from build123d import *

# Parameters (mm, degrees)
SKETCH1_W            = 15
SKETCH1_H            = 7.3
BOSS_EXTRUDE1_DEPTH  = 1
SKETCH2_W            = 3.05
SKETCH2_H            = 2.36
CUT_EXTRUDE1_DEPTH   = 1
SKETCH5_W            = 1
SKETCH5_H            = 4.94
ENGTH_EXTRUDE_DEPTH  = 1.7874
SKETCH6_W            = 4.61
SKETCH6_H            = 1
HEIGHT_EXTRUDE_DEPTH = 1.7874
SCREWS_R             = 0.5
CUT_EXTRUDE2_DEPTH   = 1
SKETCH8_W            = 1
SKETCH8_H            = 1
PINS_DEPTH           = 1


with BuildPart() as part:
    # Sketch1 → Boss-Extrude1 (new body)
    with BuildSketch(Plane.XY):
        with Locations((88.072707455, -6.376080206)):
            Rectangle(SKETCH1_W, SKETCH1_H)
    extrude(amount=BOSS_EXTRUDE1_DEPTH)

    # Sketch2 → Cut-Extrude1 (cut)
    with BuildSketch(Plane.XY.offset(1)):
        with Locations((94.047707455, -3.906080206)):
            Rectangle(SKETCH2_W, SKETCH2_H)
    extrude(amount=-CUT_EXTRUDE1_DEPTH, mode=Mode.SUBTRACT)

    # Sketch5 → :ength-Extrude (add)
    with BuildSketch(Plane(origin=(95.572707455, 0, 0), x_dir=(0, 0, -1), z_dir=(1, 0, 0))):
        with Locations((-0.5, -7.556080206)):
            Rectangle(SKETCH5_W, SKETCH5_H)
    extrude(amount=ENGTH_EXTRUDE_DEPTH)

    # Sketch6 → Height-Extrude (add)
    with BuildSketch(Plane(origin=(0, -2.726080206, 0), x_dir=(1, 0, 0), z_dir=(0, 1, 0))):
        with Locations((90.217707455, -0.5)):
            Rectangle(SKETCH6_W, SKETCH6_H)
    extrude(amount=HEIGHT_EXTRUDE_DEPTH)

    # Screws → Cut-Extrude2 (cut)
    with BuildSketch(Plane(origin=(0, 0, 0), x_dir=(-1, 0, 0), z_dir=(0, 0, -1))):
        with Locations((-81.572707455, -7.026080206)):
            Circle(SCREWS_R)
        with Locations((-88.322707455, -10.026080206)):
            Circle(SCREWS_R)
        with Locations((-94.072707455, -6.026080206)):
            Circle(SCREWS_R)
    extrude(amount=-CUT_EXTRUDE2_DEPTH, mode=Mode.SUBTRACT)

    # Sketch8 → Pins (add)
    with BuildSketch(Plane(origin=(0, 0, 0), x_dir=(-1, 0, 0), z_dir=(0, 0, -1))):
        with Locations((-92.022707455, -1.438680206)):
            Rectangle(SKETCH8_W, SKETCH8_H)
        with Locations((-88.412707455, -1.438680206)):
            Rectangle(SKETCH8_W, SKETCH8_H)
        with Locations((-96.860107455, -5.586080206)):
            Rectangle(SKETCH8_W, SKETCH8_H)
        with Locations((-96.860107455, -9.526080206)):
            Rectangle(SKETCH8_W, SKETCH8_H)
    extrude(amount=PINS_DEPTH)


solid = part.part
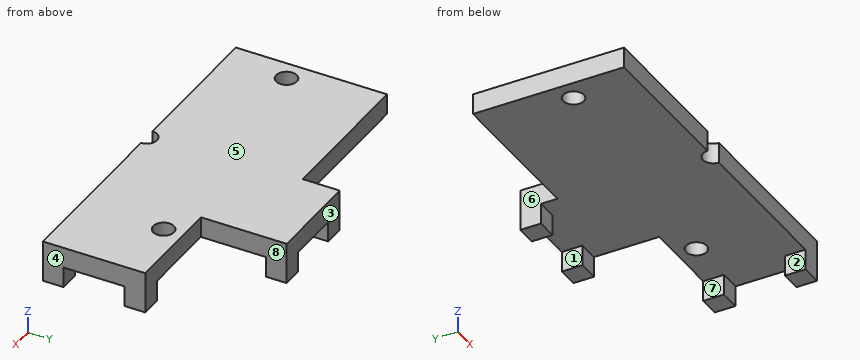
The model under review builds one solid part; all positions refer to its coordinate system, in mm. Face numbers are marked on the shaded views. A direction names the side the tool comes from. Coordinates: 2 decimals unless noted, no trailing zeros. Write each loop counter-clockwise with the first axis right and the second up, starting at its lowest first coordinate (ties: lowest second). Pieces come first, ordered by that corner, then holes. Notation, with made-up numbers: (31, -21) - (68, -21) arc R25 ccw to (68, 16) - close; hole circle Ø1 at (80, -23.75). An arc over 180 degrees is marked (long way). Answer as a JSON object with one key per item and string values. Group by question number.
1. Mouldability with a two-part tool opening along X and no side actions: class the marked faces 1, 2 and 3 as pulls with the +X half, pulls with the -X half, needs draft (parallel to the pull), parting line crosses it, or undercut.
2. Add section A-A (z = -0.3). Give the boundary of the cut face in (x, y), plus the area to 3 significant figures.
3. Add section B-B (y = -7.25). Give the boundary of the cut face in (x, z).
4. Add section D-D (x = 85). Give the boundary of the cut face in (y, z), plus the area to 3 significant figures.
5. Machinability: for the marked faces 4, 5, 6, 7 and 8, which of the approach directions +Z, -Z, +X, -X, +Y, -Y give a long, thin tool a straight path to every point of the face, cutting with its end or side? Answer none if there is none.
6. To check wall thickness, follow probe 1 along Y at (x, z) = (96.75, -0.5); probe 2 along Y at (x, z) = (86, 0.1); probe 3 along Z at (x, y) = (92.25, -3.5). State the ranges of each line that lie inside material, in increasing order.
7. Add section C-C (y = -1.5). Give the boundary of the cut face in (x, z), plus the area to 3 significant figures.
8. Clearance check with flat-ended pins moving along their axes: pin 1 Ø0.8 at (x, z) = (82.5, 0.5) entering from +Y; pin 2 Ø0.8 at (y, z) = (-5.5, -0.5) entering from -X; pin 3 Ø0.6 at (x, z) = (96, 0) entering from +Y. State where each tip first meets the part, or that it passes through.
Findings:
{
 "1": {"face 1": "undercut", "face 2": "pulls with the -X half", "face 3": "needs draft"},
 "2": {"outline": "(87.91, -1.94) - (88.91, -1.94) - (88.91, -0.94) - (87.91, -0.94) - close; (91.52, -1.94) - (92.52, -1.94) - (92.52, -0.94) - (91.52, -0.94) - close; (96.36, -10.03) - (97.36, -10.03) - (97.36, -9.03) - (96.36, -9.03) - close; (96.36, -6.09) - (97.36, -6.09) - (97.36, -5.09) - (96.36, -5.09) - close", "area": "4.00 mm²"},
 "3": {"outline": "(80.57, 0) - (81.13, 0) - (81.13, 1) - (80.57, 1) - close; (82.02, 0) - (97.36, 0) - (97.36, 1) - (82.02, 1) - close"},
 "4": {"outline": "(-10.03, 0) - (-2.73, 0) - (-2.73, 1) - (-10.03, 1) - close", "area": "7.30 mm²"},
 "5": {"face 4": "+Z, -Z, +X, +Y, -Y", "face 5": "+Z, +X, -X, +Y, -Y", "face 6": "+Z, -Z, -X, +Y", "face 7": "-Z, -X, +Y, -Y", "face 8": "+Z, -Z, +X, +Y"},
 "6": {"probe 1": "-10.03 to -9.03, -6.09 to -5.09", "probe 2": "-10.03 to -2.73", "probe 3": "0 to 1"},
 "7": {"outline": "(87.91, -1) - (88.91, -1) - (88.91, 0) - (91.52, 0) - (91.52, -1) - (92.52, -1) - (92.52, 1) - (87.91, 1) - close", "area": "6.61 mm²"},
 "8": {"pin 1": "y = -2.73", "pin 2": "x = 96.36", "pin 3": "y = -5.09"}
}
